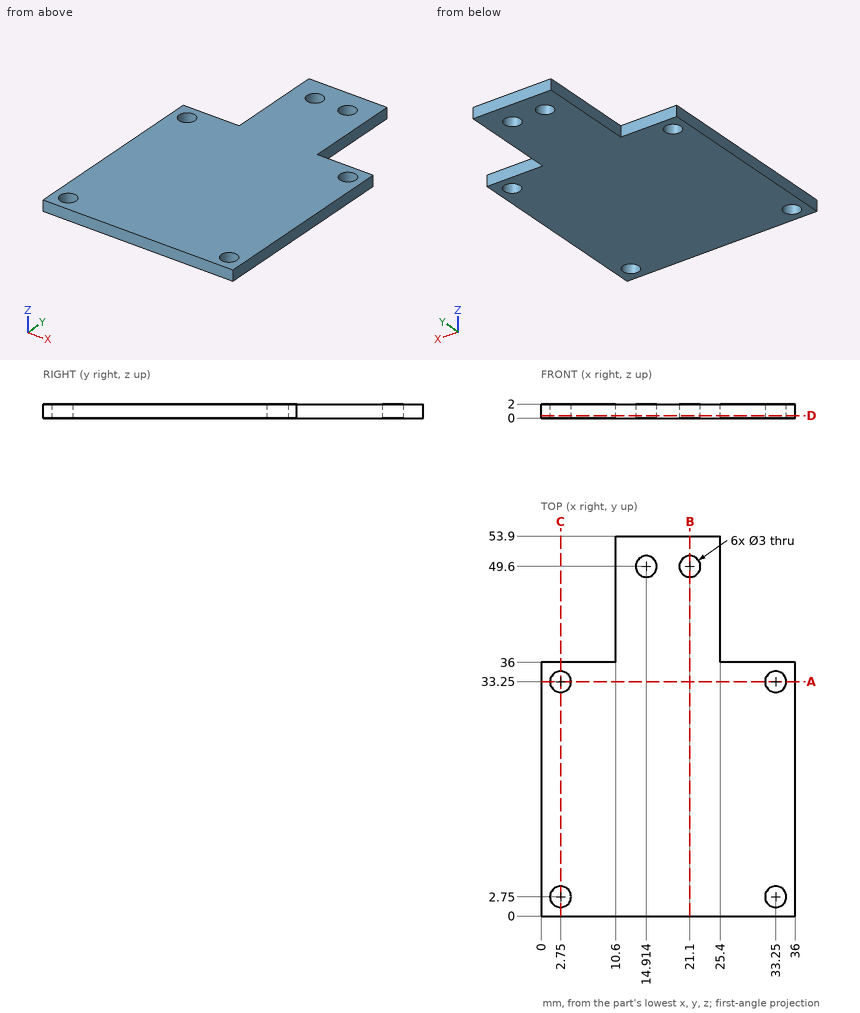
Input: dimensioned drawing with shaded views. Units: mm. Origin: part minimum x, y, z. Coordinates: 2 decimals unless noted, no trailing zeros. Loops run counter-clockwise (first coordinate to the right, second up) from the corner with the lowest first, then second, coordinate; pieces in that order, holes last. Notation, with made-up numbers: (56, -16.5) -> (112, -16.5) arc R21 cw to (112, -7.5) -> close; hole circle Ø11 at (33.5, -18). An arc over 180 degrees is marked (long way). Use a Markdown table: item, result. Add a question column.
(1) Section query B-B, the plane x = 21.1. Return loops of the section in (y, z).
(2) Section query D-D, the plane z = 0.35. Return loops of the section in (x, y).
(3) Pin query (flat end, axial travel): pin 1 Ø1 at (x, z) = (32.5, 1.5) entering from +Y; pin 2 Ø0.6 at (y, z) = (45.5, 1) entering from -X. Return the tip coordinate at first contact, or that it passes through.
(4) Line query: line 1 along Y through (x, z) = (2.75, 0.7); line 2 along Y through (x, z) = (21, 0.95); line 3 along Y through (x, z) = (2, 0.15). Output: solid intervals per line, ascending.
(5) Section query A-A, the plane y = 33.25. Return loops of the section in (x, z), plus the area to 3 significant figures.
Answer:
| question | item | result |
|---|---|---|
| 1 | outline | (0, 0) -> (48.1, 0) -> (48.1, 2) -> (0, 2) -> close; (51.1, 0) -> (53.9, 0) -> (53.9, 2) -> (51.1, 2) -> close |
| 2 | outline | (0, 0) -> (36, 0) -> (36, 36) -> (25.4, 36) -> (25.4, 53.9) -> (10.6, 53.9) -> (10.6, 36) -> (0, 36) -> close; hole circle Ø3 at (2.75, 2.75); hole circle Ø3 at (2.75, 33.25); hole circle Ø3 at (14.91, 49.6); hole circle Ø3 at (21.1, 49.6); hole circle Ø3 at (33.25, 2.75); hole circle Ø3 at (33.25, 33.25) |
| 3 | pin 1 | stops at y = 36 |
| 3 | pin 2 | stops at x = 10.6 |
| 4 | line 1 | y = 0 to 1.25, 4.25 to 31.75, 34.75 to 36 |
| 4 | line 2 | y = 0 to 48.1, 51.1 to 53.9 |
| 4 | line 3 | y = 0 to 1.45, 4.05 to 31.95, 34.55 to 36 |
| 5 | outline | (0, 0) -> (1.25, 0) -> (1.25, 2) -> (0, 2) -> close; (4.25, 0) -> (31.75, 0) -> (31.75, 2) -> (4.25, 2) -> close; (34.75, 0) -> (36, 0) -> (36, 2) -> (34.75, 2) -> close |
| 5 | area | 60.0 mm^2 |
